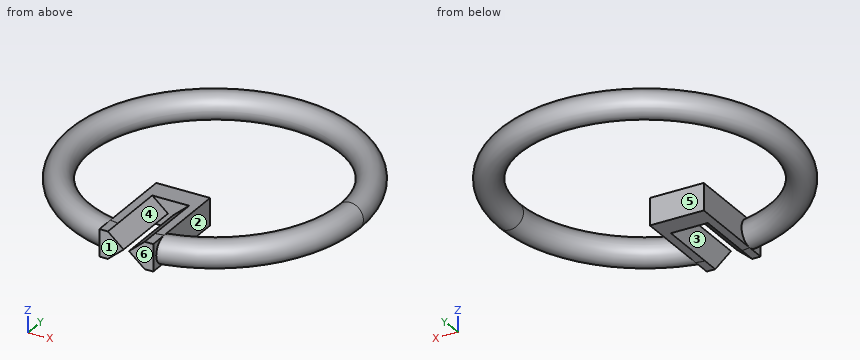
```python
from build123d import *

# Parameters (mm, degrees)
F1_R          = 2.0001698285
F4_DEPTH      = 2
F4_DEPTH_BACK = 2
F6_START      = 11.2
F6_DEPTH      = 25.6


with BuildPart() as f2:
    # F2: sweep along a path in F0
    with BuildLine(Plane.XY) as f2_path:
        CenterArc((0, 0), 18, 0, 360)
    # F1 (on Front) → F2 (sweep)
    with BuildSketch(Plane.XZ):
        with Locations((-20.043771714, 0)):
            Circle(F1_R)
    sweep(path=f2_path.line)

    # F3 (on Top) → F4 (join, two sides)
    with BuildSketch(Plane.XY) as f4_sk:
        Polygon((4, -8.0302771777), (0, -8.0302771777), (-4, -8.0302771777), (-4, -19.9341345578), (-4, -22.4341345578), (4, -22.4341345578), (4, -19.9341345578), align=None)
    extrude(amount=F4_DEPTH)
    extrude(f4_sk.sketch, amount=-F4_DEPTH_BACK)

    # F5 (on Front) → F6 (cut)
    with BuildSketch(Plane.XZ.offset(F6_START)):
        Polygon((-2.7534713777, -2.0129208903), (2.7534713777, -2.0129208903), (0.4, 0), (0, 0), (-0.4, 0), align=None)
        Polygon((0, 0), (0.4, 0), (2.7534713777, 2.0129208903), (-2.7534713777, 2.0129208903), (-0.4, 0), align=None)
    extrude(amount=F6_DEPTH, mode=Mode.SUBTRACT)


solid = f2.part
```
Verification items for the finished model (mm, model axes). Face numbers are marked on the shaded views. A direction names the side the tool comes from. Give positions to 0.01 mm unless a question says otherwise; leave off trailing zeros. Loops run counter-clockwise (first coordinate to the right, second up) from the corner with the lowest first, then second, coordinate; pieces in that order, holes last.
1. Thickness scan on line 1 (X direction, y = -15, z = -1.15); line 2 (X direction, y = 4.5, z = -1.6); line 3 (Y direction, x = -9, z = -0.5). Record the ranges inside material, lowest first.
2. Section check B-B, the plane y = -9. Count the separate pieces of the cut face and the enclosed holes in it, then the cut area to 3 significant figures.
3. Go/stop test with flat-tipped pins: pin 1 Ø2 at (y, z) = (-16.5, 0.5) entering from -X; pin 2 Ø1.4 at (y, z) = (-20.5, 0.5) entering from +X; pin 3 Ø2 at (y, z) = (-15, 0) entering from +X. Record where each tip stops, or that it passes through.
4. Section check A-A, the plane z = -1.05. Enter the section's corners in (x, y), then the cut area to 3 significant figures.
5. Set-up check for the marked faces 4, 5 and 6: record each of +Z, -Z, +X, -X, +Y, -Y from which the full face is reachable in a straight line by a thin tool's end or side.
6. Mould release check, pull along X, two halves, no side actions. Record for the marked faces 1, 2 and 3: released by +X, released by -X, zero draft, split by the parting line, or undercut.
Geometry says:
1. line 1: x = -15.65 to -10.67, -4 to -1.74, 1.74 to 4, 10.67 to 15.65
1. line 2: x = -20.76 to -18.3, 18.3 to 20.76
1. line 3: y = -20.05 to -15.71, 15.71 to 20.05
2. separate pieces: 3
2. enclosed holes: 0
2. area: 60.2 mm2
3. pin 1: stops at x = -15.62
3. pin 2: stops at x = 9.59
3. pin 3: stops at x = 17.03
4. outline: (-4, -22.43) - (-1.63, -22.43) - (-1.63, -11.2) - (1.63, -11.2) - (1.63, -22.43) - (4, -22.43) - (4, -21.38) arc R21.75 ccw (long way) to (-4, -21.38) - close; hole (-4, -17.9) - (-4, -8.03) - (4, -8.03) - (4, -17.9) arc R18.34 ccw (long way) to start
4. area: 480 mm2
5. face 4: +Z, -Y
5. face 5: +Z, -Z
5. face 6: +Z, -Z, +X, -X, -Y
6. face 1: zero draft
6. face 2: undercut
6. face 3: undercut
